The listing builds one solid part. Answer for the finished solid, in the listing's coordinates (mm). Face numbers are marked on the shaded views. A direction names the side the tool comes from. Round coordinates to 2 decimals unless told otherwise and drop trailing zeros. Loops run counter-clockwise (first coordinate to the right, second up) from the corner with the lowest first, then second, coordinate; pieces in that order, holes last. Notation, with made-up numbers: (70.25, 22) -> (83.25, 22) arc R16 ccw to (83.25, 40) -> close; hole circle Ø8 at (74.25, 23.25). An arc over 180 degrees is marked (long way). Use a Markdown table: item, result. Add a question column.
Q1. Section D-D on x = 15.24 is taken. Give the vertices of the cut face in (y, z) (3 decimals), then the cut area to 3 significant figures.
Q2. Section A-A on y = 0 is taken. Give the vertices of the cut face in (x, z) (3 decimals), then the cut area to 3 significant figures.
Q3. Section C-C on y = 8 is taken. Give the vertices of the cut face in (x, z) (1 decimal).
Q4. Given pin 1 Ø1.5 at (y, z) = (-7.5, 1.5) entering from -X; pin 2 Ø2 at (x, y) = (10, 7.5) entering from -Z (3 decimals); pin 3 Ø2 at (x, z) = (7.5, 2) entering from +Y, each flat-ended and moving along its own axis, determine where each tip first touches the part or whether it passes through.
Q5. For a pull along X with two mould halves and no side action, classify the marked faces 1, 2, 3 and 4 as released by +X, released by -X, zero draft, split by the parting line, or undercut.
Q6. Consider line 1 (Y direction, x = 0, z = 3.5) (3 decimals); line 2 (X direction, y = 1, z = 6.5); line 3 (Y direction, x = 0.5, z = 6.5). Determine where each line is inside the solid, lowest interval first.
Q7. Which of the six approach directions +Z, -Z, +X, -X, +Y, -Y give full straight-line access (tool end or side, diameter ignored) to the marked faces 5 and 6?
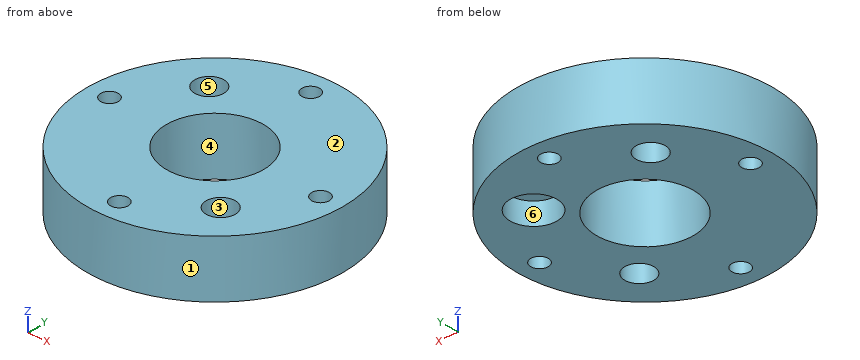
Autodesk Inventor part; units mm, degrees
ref_plane "YZ Plane" through (0, 0, 0) normal (1, 0, 0) x (0, 1, 0)
ref_plane "XZ Plane" through (0, 0, 0) normal (0, 1, 0) x (-1, 0, 0)
ref_plane "XY Plane" through (0, 0, 0) normal (0, 0, 1) x (1, 0, 0)
sketch "Sketch7" plane through (0, 0, 0) normal (0, 0, 1) x (1, 0, 0)
  line L0 (0, 0) -> (0, 15.24)
  circle A0 centre (0, 15.24) radius 1.27
  circle A1 centre (-15.24, 0) radius 1.27
  circle A2 centre (0, -15.24) radius 1.27
  circle A3 centre (15.24, 0) radius 1.27
  circle A4 centre (0, 0) radius 18.415
  line L1 (0, 0) -> (8.4414, 8.4414)
  line L2 (0, 0) -> (11.938, 0) construction
  circle A5 centre (8.4414, 8.4414) radius 3.3655
  dimension "d82" = 15.24
  dimension "d83" = 2.54
  dimension "d86" = 360
  dimension "d88" = 36.83
  dimension "d89" = 11.938
  dimension "d90" = 45
  dimension "d91" = 6.731
extrude "Extrusion8" add sketch "Sketch7" along normal blind 8.255
sketch "Sketch8" plane through (0, 0, 8.255) normal (0, 0, 1) x (1, 0, 0)
  circle A0 centre (0, 0) radius 6.985
  dimension "d94" = 13.97
extrude "Extrusion9" cut sketch "Sketch8" against normal through all
sketch "Sketch10" plane through (0, 0, 8.255) normal (0, 0, 1) x (1, 0, 0)
  circle A0 centre (8.4414, 8.4414) radius 3.3655
  point P0 (0, 0)
extrude "Extrusion10" add sketch "Sketch10" against normal blind 5.08
sketch "Sketch11" plane through (0, 0, 8.255) normal (0, 0, 1) x (1, 0, 0)
  line L0 (0, 0) -> (-8.8388, 8.8388)
  line L1 (0, 0) -> (12.5, 0) construction
  line L2 (0, 0) -> (8.8388, -8.8388)
  circle A0 centre (-8.8388, 8.8388) radius 2.0955
  circle A1 centre (8.8388, -8.8388) radius 2.0955
  dimension "d99" = 12.5
  dimension "d100" = 135
  dimension "d101" = 12.5
  dimension "d102" = 4.191
  dimension "d103" = 4.191
extrude "Extrusion11" cut sketch "Sketch11" against normal through all
equation "\"d101\" = d99"
equation "\"d102\" = d103"
properties part number "idlerShaftBearingMount" material "ABS Plastic"
Checked values:
| question | item | result |
|---|---|---|
| 1 | outline | (-10.337, 0) -> (-1.27, 0) -> (-1.27, 8.255) -> (-10.337, 8.255) -> close; (1.27, 0) -> (10.337, 0) -> (10.337, 8.255) -> (1.27, 8.255) -> close |
| 1 | area | 150 mm2 |
| 2 | outline | (-18.415, 0) -> (-16.51, 0) -> (-16.51, 8.255) -> (-18.415, 8.255) -> close; (-13.97, 0) -> (-6.985, 0) -> (-6.985, 8.255) -> (-13.97, 8.255) -> close; (6.985, 0) -> (13.97, 0) -> (13.97, 8.255) -> (6.985, 8.255) -> close; (16.51, 0) -> (18.415, 0) -> (18.415, 8.255) -> (16.51, 8.255) -> close |
| 2 | area | 147 mm2 |
| 3 | outline | (-16.6, 0) -> (-10.8, 0) -> (-10.8, 8.3) -> (-16.6, 8.3) -> close; (-6.9, 0) -> (5.1, 0) -> (5.1, 3.2) -> (11.8, 3.2) -> (11.8, 0) -> (16.6, 0) -> (16.6, 8.3) -> (-6.9, 8.3) -> close |
| 4 | pin 1 | stops at x = -17.13 |
| 4 | pin 2 | stops at z = 3.175 |
| 4 | pin 3 | stops at y = 17.23 |
| 5 | face 1 | split by the parting line |
| 5 | face 2 | zero draft |
| 5 | face 3 | undercut |
| 5 | face 4 | undercut |
| 6 | line 1 | y = -18.415 to -16.51, -13.97 to -6.985, 6.985 to 13.97, 16.51 to 18.415 |
| 6 | line 2 | x = -18.39 to -16.02, -14.46 to -6.91, 6.91 to 14.46, 16.02 to 18.39 |
| 6 | line 3 | y = -18.41 to -16.41, -14.07 to -6.97, 6.97 to 14.07, 16.41 to 18.41 |
| 7 | face 5 | +Z, -Z |
| 7 | face 6 | -Z |
